Check sheet for the modelled part. Datum: model origin and axes. Units: mm. A direction names the side the tool comes from. Round coordinates to 2 decimals unless told otherwise and drop trailing zeros. Write each loop counter-clockwise with the first axis right and the second up, starting at its lowest first coordinate (ties: lowest second). Pieces come first, ordered by that corner, then holes. Notation, with made-up numbers: (54, 25.5) -> (73, 25.5) arc R29 cw to (73, 51.5) -> close; hole circle Ø4 at (42.25, 47). An arc over 180 degrees is marked (long way). One line per item, written item: value.
from build123d import *

# Parameters (mm, degrees)
SKICA1_R                 = 5
SKICA1_R_2               = 4
P_IDAT_VYSUNUT_M1_DEPTH  = 8
SKICA2_R                 = 11
SKICA2_R_2               = 4
P_IDAT_VYSUNUT_M2_DEPTH  = 3
SKICA3_R                 = 1.5
ODEBRAT_VYSUNUT_M3_DEPTH = 3


with BuildPart() as part:
    # Skica1 → Přidat vysunutím1 (new body)
    with BuildSketch(Plane(origin=(0, 0, 0), x_dir=(1, 0, 0), z_dir=(0, 1, 0))):
        with Locations(Location((0, 0, 0), (0, 0, 270))):
            Circle(SKICA1_R)
        with Locations(Location((0, 0, 0), (0, 0, 270))):
            Circle(SKICA1_R_2, mode=Mode.SUBTRACT)
    extrude(amount=P_IDAT_VYSUNUT_M1_DEPTH)

    # Skica2 → Přidat vysunutím2 (add)
    with BuildSketch(Plane(origin=(0, 8, 0), x_dir=(1, 0, 0), z_dir=(0, 1, 0))):
        with Locations(Location((0, 0, 0), (0, 0, 270))):
            Circle(SKICA2_R)
        with Locations(Location((0, 0, 0), (0, 0, 270))):
            Circle(SKICA2_R_2, mode=Mode.SUBTRACT)
    extrude(amount=P_IDAT_VYSUNUT_M2_DEPTH)

    # Skica3 → Odebrat vysunutím3 (cut)
    with BuildSketch(Plane(origin=(0, 11, 0), x_dir=(1, 0, 0), z_dir=(0, 1, 0))):
        with Locations(Location((8, 0, 0), (0, 0, 270))):
            Circle(SKICA3_R)
        with Locations(Location((-8, 0, 0), (0, 0, 270))):
            Circle(SKICA3_R)
    extrude(amount=-ODEBRAT_VYSUNUT_M3_DEPTH, mode=Mode.SUBTRACT)


solid = part.part
Item 1: Sectioned sample at B-B on z = 0. Enter the section's corners in (x, y), and give its area (3 significant figures).
Answer:
outline: (-11, 8) -> (-9.5, 8) -> (-9.5, 11) -> (-11, 11) -> close; (-6.5, 8) -> (-5, 8) -> (-5, 0) -> (-4, 0) -> (-4, 11) -> (-6.5, 11) -> close; (4, 0) -> (5, 0) -> (5, 8) -> (6.5, 8) -> (6.5, 11) -> (4, 11) -> close; (9.5, 8) -> (11, 8) -> (11, 11) -> (9.5, 11) -> close
area: 40.0 mm^2
Item 2: Thickness scan on line 1 (X direction, y = 10.35, z = 0); line 2 (X direction, y = 6, z = 0); line 3 (Y direction, x = -6.5, z = 3.75). Record the ranges inside material, lowest first.
Answer:
line 1: x = -11 to -9.5, -6.5 to -4, 4 to 6.5, 9.5 to 11
line 2: x = -5 to -4, 4 to 5
line 3: y = 8 to 11
Item 3: Tool access check on faces 1 (the flat face through (-5, 11, 0)), 2 (the cylindrical face through (-4.88, 3.94, -1.08)). Record the directions out of +Z, -Z, +X, -X, +Y, -Y that give a thin tool (end or side, any length) a straight path to the whole face; none if there is none.
Answer:
face 1: +Z, -Z, +X, -X, +Y
face 2: -Y
Item 4: Sectioned sample at A-A on x = 0. Enter the section's corners in (y, z).
Answer:
outline: (0, -5) -> (8, -5) -> (8, -11) -> (11, -11) -> (11, -4) -> (0, -4) -> close; (0, 4) -> (11, 4) -> (11, 11) -> (8, 11) -> (8, 5) -> (0, 5) -> close
Item 5: Depth check by flat-ended pin: P1, Ø8, axis at x = 7, z = -7, coming from the -Y side; P2, Ø3, axis at x = 7.5, y = 3, coming from the -Z side. Enter the tip coordinate at first touch or a pass-through.
Answer:
P1: stops at y = 8
P2: passes through
Item 6: Sectioned sample at D-D on z = -2.5. Enter the section's corners in (x, y).
Answer:
outline: (-10.71, 8) -> (-4.33, 8) -> (-4.33, 0) -> (-3.12, 0) -> (-3.12, 11) -> (-10.71, 11) -> close; (3.12, 0) -> (4.33, 0) -> (4.33, 8) -> (10.71, 8) -> (10.71, 11) -> (3.12, 11) -> close
Item 7: Sectioned sample at C-C on y = 5. Enter the section's corners in (x, z).
Answer:
outline: circle Ø10 at (0, 0); hole circle Ø8 at (0, 0)
